Input: dimensioned drawing with shaded views. Units: mm. Origin: part minimum x, y, z. A direction names the side the tool comes from. Give positions to 0.01 mm unless a question says otherwise; leave off trailing zeros. Order: outer loops, then holes, each group sorted by start corner. A loop starts at its lowest first (then second) coordinate and runs counter-clockwise, first axis right, second up. Notation, with made-up numbers: (84.5, 70.5) - (91.5, 70.5) arc R26 ccw to (91.5, 91.5) - close; hole circle Ø10 at (-30.5, -36). An arc over 180 degrees is marked (long way). Answer as CSV lines item,"result".
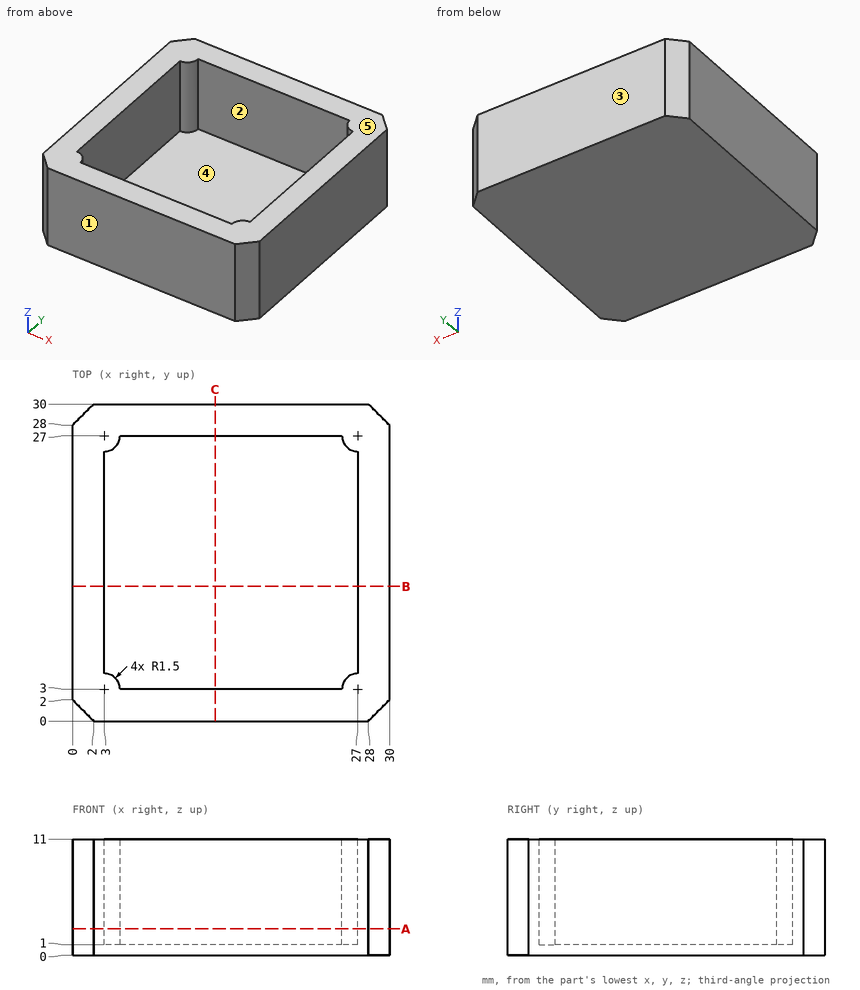
(1) Cut plane A-A (z = 2.5). Return loops of the section in (x, y).
Completed:
outline,"(0, 2) - (2, 0) - (28, 0) - (30, 2) - (30, 28) - (28, 30) - (2, 30) - (0, 28) - close; hole (3, 4.5) arc R1.5 cw to (4.5, 3) - (25.5, 3) arc R1.5 cw to (27, 4.5) - (27, 25.5) arc R1.5 cw to (25.5, 27) - (4.5, 27) arc R1.5 cw to (3, 25.5) - close"
(2) Contact query for a flat-ended pin moving along its axis: pin 1 (1 mm diameter, centred on x = 8, y = 20.5, fed in from +Z). Output: stop coordinate, or through.
Completed:
pin 1,"z = 1"
(3) Cut plane B-B (y = 12.75). Return loops of the section in (x, z).
Completed:
outline,"(0, 0) - (30, 0) - (30, 11) - (27, 11) - (27, 1) - (3, 1) - (3, 11) - (0, 11) - close"
(4) Mould query, pull axis Y, two halves, no side actions, for the marked faces 1, 2 and 3. Classes: released by +Y, released by -Y, zero draft, split by the parting line, or undercut.
Completed:
face 1,"released by -Y"
face 2,"undercut"
face 3,"released by +Y"
(5) Access query for the marked faces 4 and 5. Directions: +Z, -Z, +X, -X, +Y, -Y. A direction counts if a zero-diameter tool reaches every point of the face in a straight line with its end or side. Return the directions, or none.
Completed:
face 4,"+Z"
face 5,"+Z, +X, -X, +Y, -Y"
(6) Ray query, line 1 (Y direction, x = 16.75, z = 4); line 2 (Z direction, x = 25, y = 19.5). Return the intervals inside material, ascending. Write a range as from..to.
Completed:
line 1,"0..3, 27..30"
line 2,"0..1"
